Read the model definition and answer for the solid it produces. Units are mm, in the model's axes. Face numbers are marked on the shaded views. A direction names the side the tool comes from. Give positions to 0.01 mm unless a question says otherwise; leave off trailing zeros. Order: outer loops, then holes, each group sorted by start corner. A loop starts at its lowest first (then second) coordinate and runs counter-clockwise, first axis right, second up. Notation, with made-up numbers: (-40, 29.5) -> (-36, 29.5) arc R30 ccw to (-36, 58.5) -> close; hole circle Ø5 at (9.25, 31.5). An arc over 180 degrees is marked (long way). One line per item, written item: value. Start each with the question number.
Autodesk Inventor part; units mm, degrees
ref_plane "dummy_to_bolt_XY" through (0, 0, 0) normal (1, 0, 0) x (0, 0, -1)
ref_plane "dummy_to_bolt_YZ" through (0, 0, 0) normal (0, 0, -1) x (0, 1, 0)
ref_plane "dummy_to_bolt_ZX" through (0, 0, 0) normal (0, 1, 0) x (1, 0, 0)
sketch "Sketch_1" plane through (0, 0, 0) normal (0, 0, 1) x (1, 0, 0)
  line L0 (4.3, 0) -> (0, 0)
  line L1 (-1.7, 0) -> (-1.7, 3)
  line L2 (-1.7, 3) -> (-1.5, 3)
  line L3 (-1.5, 3) -> (0, 1.5)
  line L4 (0, 1.5) -> (3.9935, 1.5)
  line L5 (3.9935, 1.5) -> (4.3, 1.1935)
  line L6 (4.3, 1.1935) -> (4.3, 0)
  line L7 (4.3, 0) -> (-1.7, 0)
revolve "Revolution1" add sketch "Sketch_1" angle 360 about axis through (4.3, 0, 0) along (1, 0, 0)
thread "Thread1"
sketch "Sketch_4" plane through (0, 0, 0) normal (0, 0, 1) x (1, 0, 0)
  line L0 (-0.5821, 0) -> (-1.7, 0)
  line L1 (-1.7, 0) -> (-1.7, 1)
  line L2 (-1.7, 1) -> (-0.85, 1)
  line L3 (-0.85, 1) -> (-0.5821, 0)
  line L4 (-0.5821, 0) -> (-1.7, 0)
revolve "Revolution2" cut sketch "Sketch_4" angle 360 about axis through (-0.5821, 0, 0) along (1, 0, 0)
sketch "Sketch_3" plane through (-1.7, 0, 0) normal (1, 0, 0) x (0, 0, -1)
  line L0 (-1, 0.5774) -> (-1, -0.5774)
  line L1 (-1, -0.5774) -> (0, -1.1547)
  line L2 (0, -1.1547) -> (1, -0.5774)
  line L3 (1, -0.5774) -> (1, 0.5774)
  line L4 (1, 0.5774) -> (0, 1.1547)
  line L5 (0, 1.1547) -> (-1, 0.5774)
extrude "Extrusion1" cut sketch "Sketch_3" along normal blind 0.85
ref_plane "dummy_to_bolt_XY" through (0, 0, 0) normal (1, 0, 0) x (0, 0, -1)
ref_plane "dummy_to_bolt_YZ" through (0, 0, 0) normal (0, 0, -1) x (0, 1, 0)
ref_plane "dummy_to_bolt_ZX" through (0, 0, 0) normal (0, 1, 0) x (1, 0, 0)
ref_plane "bolt_to_nut_XY" through (4.3, 0, 0) normal (1, 0, 0) x (0, 0, -1)
ref_plane "bolt_to_nut_YZ" through (4.3, 0, 0) normal (0, 0, -1) x (0, 1, 0)
ref_plane "bolt_to_nut_ZX" through (4.3, 0, 0) normal (0, 1, 0) x (1, 0, 0)
properties part number "HFBCM3-6"
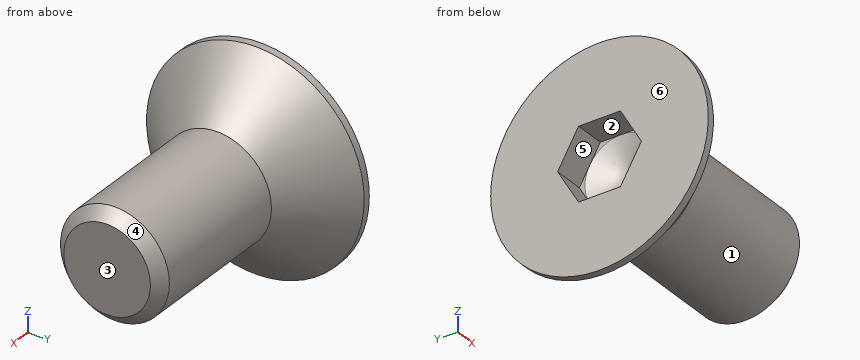
Item 1: Flat-ended cylindrical pins translate along their axes: pin 1 (0.9 mm diameter, centred on x = -1, y = 0, fed in from +Z); pin 2 (3 mm diameter, centred on x = 0.5, z = 1.5, fed in from +Y); pin 3 (0.7 mm diameter, centred on x = -1, y = 0, fed in from -Z). Find the tip coordinate at first contact, or state that the pin passes through.
Item 2: For a pull along Y with two mould halves and no side action, classify the marked faces 4, 5 and 6 as +Y half, -Y half, draft (parallel to the pull), parting line (faces both ways), or undercut.
Item 3: Find section A-A on x = 0.4. Write down the section's boundary in (y, z).
Item 4: Find the intervals of material crossed by line 1 (Z direction, x = -1.15, y = -1.1); line 2 (Y direction, x = 0.8, z = -1); line 3 (X direction, y = -1.2, z = 1.05), in increasing order. Write a range as from..to.
Item 5: A tool of negligible diameter and unlimited length cuts with its end or side. For the marked faces 1, 2 and 3, from which of +Z, -Z, +X, -X, +Y, -Y can it reach the whole face along a straight path? Write none if from no direction.
Checks:
1. pin 1: z = 2.95
1. pin 2: y = 2.2
1. pin 3: z = -2.85
2. face 4: parting line
2. face 5: undercut
2. face 6: draft
3. outline: circle Ø3 at (0, 0)
4. line 1: -2.41..-0.09, 0.09..2.41
4. line 2: -1.12..1.12
4. line 3: -1.7..-0.09
5. face 1: +X
5. face 2: -X
5. face 3: +Z, -Z, +X, +Y, -Y
